from build123d import *

# Parameters (mm, degrees)
SKETCH_1_W               = 165.5
SKETCH_1_H               = 60
EXTRUDE_1_DEPTH          = 4
EXTRUDE_2_DEPTH          = 4
SKETCH_3_W               = 214.285714285
SKETCH_3_H               = 25
EXTRUDE_5_DEPTH          = 4
SKETCH_4_R               = 2.75
CUT_EXTRUDE_1_DEPTH      = 4
SKETCH_5_W               = 55
SKETCH_5_H               = 20
CUT_EXTRUDE_2_DEPTH      = 4
FILLET_1_R               = 10
SKETCH_6_W               = 186.285714285
SKETCH_6_H               = 14
CUT_EXTRUDE_3_DEPTH      = 4
SKETCH_7_R               = 1.5
CUT_EXTRUDE_4_DEPTH      = 4
FILLET_2_R               = 3
CUT_EXTRUDE_5_DEPTH      = 4
FILLET_1_OF_MIRROR_1_R   = 10
FILLET_2_OF_MIRROR_1_R   = 3
CUT_EXTRUDE_6_DEPTH      = 292.712781796
CUT_EXTRUDE_6_DEPTH_BACK = 4
SKETCH_9_W               = 205.055051827
SKETCH_9_H               = 163.821453507
CUT_EXTRUDE_7_DEPTH      = 293.240221501
SKETCH_11_W              = 207.248718004
SKETCH_11_H              = 34
EXTRUDE_6_DEPTH          = 4
SKETCH_12_W              = 22
SKETCH_12_H              = 28
EXTRUDE_7_DEPTH          = 4
SKETCH_13_R              = 2.75
CUT_EXTRUDE_8_DEPTH      = 4
EXTRUDE_8_DEPTH          = 4
FILLET_3_R               = 10
SKETCH_15_W              = 10
SKETCH_15_H              = 10
CUT_EXTRUDE_9_DEPTH      = 4
FILLET_4_R               = 2
CHAMFER_1_SIZE           = 0.5
CHAMFER_2_SIZE           = 0.5


with BuildPart() as part:
    # 草图1 → 凸台-拉伸1 (new body)
    with BuildSketch(Plane(origin=(0, 0, 0), x_dir=(0, 0, -1), z_dir=(1, 0, 0))):
        with Locations((82.75, 30)):
            Rectangle(SKETCH_1_W, SKETCH_1_H)
    extrude_1 = extrude(amount=EXTRUDE_1_DEPTH)

    # 草图2 → 凸台-拉伸2 (add)
    with BuildSketch(Plane(origin=(0, 0, -165.5), x_dir=(-1, 0, 0), z_dir=(0, 0, -1))):
        Polygon((-4, 30), (-204, 106.930925816), (-193.94769236, 133.06425915), (-4, 60), align=None)
    extrude_2 = extrude(amount=-EXTRUDE_2_DEPTH)

    # 草图3 → 凸台-拉伸5 (add)
    with BuildSketch(Plane(origin=(-9.536752084, 24.793025648, 0), x_dir=(0.9333333333333335, 0.3590109871422999, 0), z_dir=(0.3590109871422999, -0.9333333333333335, 0))):
        with Locations((121.646520091, -153)):
            Rectangle(SKETCH_3_W, SKETCH_3_H)
    extrude_5 = extrude(amount=-EXTRUDE_5_DEPTH)

    # 草图4 → 切除-拉伸1 (cut)
    with BuildSketch(Plane(origin=(4, 0, 0), x_dir=(0, 0, -1), z_dir=(1, 0, 0))):
        with Locations((50, 50)):
            Circle(SKETCH_4_R)
        with Locations((50, 20)):
            Circle(SKETCH_4_R)
    cut_extrude_1 = extrude(amount=-CUT_EXTRUDE_1_DEPTH, mode=Mode.SUBTRACT)

    # 草图5 → 切除-拉伸2 (cut)
    with BuildSketch(Plane(origin=(4, 0, 0), x_dir=(0, 0, -1), z_dir=(1, 0, 0))):
        with Locations((138, 10)):
            Rectangle(SKETCH_5_W, SKETCH_5_H)
    cut_extrude_2 = extrude(amount=-CUT_EXTRUDE_2_DEPTH, mode=Mode.SUBTRACT)

    # 圆角1
    fillet_1_edges = [part.edges().sort_by_distance(p)[0] for p in [
        (2, 20, -165.5),
        (2, 20, -110.5),
        (2, 0, -110.5),
    ]]
    fillet(fillet_1_edges, radius=FILLET_1_R - 0.0001)  # a hair under: the kernel refuses the full size

    # 草图6 → 切除-拉伸3 (cut)
    with BuildSketch(Plane(origin=(-9.536752084, 24.793025648, 0), x_dir=(0.9333333333333335, 0.35901098714229984, 0), z_dir=(0.35901098714229984, -0.9333333333333335, 0))):
        with Locations((121.646520091, -147.5)):
            Rectangle(SKETCH_6_W, SKETCH_6_H)
    cut_extrude_3 = extrude(amount=-CUT_EXTRUDE_3_DEPTH, mode=Mode.SUBTRACT)

    # 草图7 → 切除-拉伸4 (cut)
    with BuildSketch(Plane(origin=(-9.536752084, 24.793025648, 0), x_dir=(0.9333333333333335, 0.35901098714229984, 0), z_dir=(0.35901098714229984, -0.9333333333333335, 0))):
        with Locations((221.789377233, -145.5)):
            Circle(SKETCH_7_R)
        with Locations((21.789377233, -145.5)):
            Circle(SKETCH_7_R)
    cut_extrude_4 = extrude(amount=-CUT_EXTRUDE_4_DEPTH, mode=Mode.SUBTRACT)

    # 圆角2
    fillet_2_edges = [part.edges().sort_by_distance(p)[0] for p in [
        (4, 32.142857143, -140.5),
        (203.281978026, 108.797592483, -140.5),
        (16.348644692, 36.892820487, -140.5),
        (190.215311359, 103.771438663, -140.5),
    ]]
    fillet(fillet_2_edges, radius=FILLET_2_R)

    # 草图8 → 切除-拉伸5 (cut)
    with BuildSketch(Plane.XY.offset(-161.5)):
        Polygon((45.333333333, 45.899058002), (39.948168526, 59.899058002), (170.614835193, 110.160596202), (176, 96.160596202), align=None)
    cut_extrude_5 = extrude(amount=-CUT_EXTRUDE_5_DEPTH, mode=Mode.SUBTRACT)

    # 镜向1: 凸台-拉伸1, 凸台-拉伸2, 凸台-拉伸5, 切除-拉伸1, 切除-拉伸2, 切除-拉伸3, 切除-拉伸4, 切除-拉伸5 across plane
    add(extrude_1.mirror(Plane.XY))
    add(extrude_2.mirror(Plane.XY))
    add(extrude_5.mirror(Plane.XY))
    add(cut_extrude_1.mirror(Plane.XY), mode=Mode.SUBTRACT)
    add(cut_extrude_2.mirror(Plane.XY), mode=Mode.SUBTRACT)
    add(cut_extrude_3.mirror(Plane.XY), mode=Mode.SUBTRACT)
    add(cut_extrude_4.mirror(Plane.XY), mode=Mode.SUBTRACT)
    add(cut_extrude_5.mirror(Plane.XY), mode=Mode.SUBTRACT)

    # 圆角1 of 镜向1
    fillet_1_of_mirror_1_edges = [part.edges().sort_by_distance(p)[0] for p in [
        (2, 20, 165.5),
        (2, 20, 110.5),
        (2, 0, 110.5),
    ]]
    fillet(fillet_1_of_mirror_1_edges, radius=FILLET_1_OF_MIRROR_1_R - 0.0001)  # a hair under: the kernel refuses the full size

    # 圆角2 of 镜向1
    fillet_2_of_mirror_1_edges = [part.edges().sort_by_distance(p)[0] for p in [
        (4, 32.142857143, 140.5),
        (203.281978026, 108.797592483, 140.5),
        (16.348644692, 36.892820487, 140.5),
        (190.215311359, 103.771438663, 140.5),
    ]]
    fillet(fillet_2_of_mirror_1_edges, radius=FILLET_2_OF_MIRROR_1_R)

    # 草图9 → 切除-拉伸6 (cut, two sides: drawn at the far end of the back side and taken through both)
    with BuildSketch(Plane(origin=(4, 0, 0), x_dir=(0, 0, -1), z_dir=(1, 0, 0)).offset(-CUT_EXTRUDE_6_DEPTH_BACK)):
        with Locations((102.527525913, 81.910726754)):
            Rectangle(SKETCH_9_W, SKETCH_9_H)
    extrude(amount=CUT_EXTRUDE_6_DEPTH + CUT_EXTRUDE_6_DEPTH_BACK, mode=Mode.SUBTRACT)

    # 草图10 → 切除-拉伸7 (cut, through all)
    with BuildSketch(Plane.XY.offset(161.5)):
        Polygon((174.563956051, 99.893929535), (43.897289385, 49.632391335), (45.333333333, 45.899058002), (176, 96.160596202), align=None)
    extrude(amount=-CUT_EXTRUDE_7_DEPTH, mode=Mode.SUBTRACT)

    # 草图11 → 凸台-拉伸6 (add)
    with BuildSketch(Plane(origin=(-19.589059724, 50.926358981, 0), x_dir=(0.9333333333333335, 0.3590109871422999, 0), z_dir=(-0.3590109871422999, 0.9333333333333335, 0))):
        with Locations((125.165018231, -148.5)):
            Rectangle(SKETCH_11_W, SKETCH_11_H)
    extrude(amount=-EXTRUDE_6_DEPTH)

    # 草图12 → 凸台-拉伸7 (add)
    with BuildSketch(Plane(origin=(213.536752084, 82.137900168, 0), x_dir=(0, 0, -1), z_dir=(0.9333333333333338, 0.35901098714229945, 0))):
        with Locations((-154.5, 40.563956051)):
            Rectangle(SKETCH_12_W, SKETCH_12_H)
    extrude(amount=EXTRUDE_7_DEPTH)

    # 草图13 → 切除-拉伸8 (cut)
    with BuildSketch(Plane(origin=(217.270085418, 83.573944117, 0), x_dir=(0, 0, -1), z_dir=(0.9333333333333338, 0.35901098714229945, 0))):
        with Locations(Location((-155.5, 40.563956051, 0), (0, 0, 90))):
            Circle(SKETCH_13_R)
    extrude(amount=-CUT_EXTRUDE_8_DEPTH, mode=Mode.SUBTRACT)

    # 草图14 → 凸台-拉伸8 (add)
    with BuildSketch(Plane(origin=(0, 0, 131.5), x_dir=(-1, 0, 0), z_dir=(0, 0, -1))):
        Polygon((-4, 55.714285714), (-4, 60), (0, 60), (0, 133.06425915), (-193.94769236, 133.06425915), (-195.383736309, 129.330925816), align=None)
    extrude(amount=EXTRUDE_8_DEPTH)

    # 圆角3
    fillet_3_edges = [part.edges().sort_by_distance(p)[0] for p in [
        (0, 133.06425915, 129.5),
    ]]
    fillet(fillet_3_edges, radius=FILLET_3_R)

    # 草图15 → 切除-拉伸9 (cut)
    with BuildSketch(Plane.XY.offset(131.5)):
        with Locations((15, 118.06425915)):
            Rectangle(SKETCH_15_W, SKETCH_15_H)
        with Locations((27, 118.06425915)):
            Rectangle(SKETCH_15_W, SKETCH_15_H)
        with Locations((15, 106.06425915)):
            Rectangle(SKETCH_15_W, SKETCH_15_H)
        with Locations((27, 106.06425915)):
            Rectangle(SKETCH_15_W, SKETCH_15_H)
    extrude(amount=-CUT_EXTRUDE_9_DEPTH, mode=Mode.SUBTRACT)

    # 圆角4
    fillet_4_edges = [part.edges().sort_by_distance(p)[0] for p in [
        (32, 123.06425915, 129.5),
        (10, 101.06425915, 129.5),
        (32, 101.06425915, 129.5),
        (10, 123.06425915, 129.5),
    ]]
    fillet(fillet_4_edges, radius=FILLET_4_R)

    # 倒角1
    chamfer_1_edges = [part.edges().sort_by_distance(p)[0] for p in [
        (22, 118.06425915, 127.5),
        (22, 113.06425915, 129.5),
        (22, 123.06425915, 129.5),
        (32, 117.06425915, 127.5),
        (27, 113.06425915, 127.5),
        (22, 118.06425915, 131.5),
        (27, 113.06425915, 131.5),
        (32, 117.06425915, 131.5),
        (10, 107.06425915, 127.5),
        (15, 111.06425915, 127.5),
        (10, 111.06425915, 129.5),
        (10, 107.06425915, 131.5),
        (15, 111.06425915, 131.5),
        (22, 106.06425915, 127.5),
        (22, 101.06425915, 129.5),
        (27, 111.06425915, 127.5),
        (22, 111.06425915, 129.5),
        (26, 101.06425915, 127.5),
        (22, 106.06425915, 131.5),
        (26, 101.06425915, 131.5),
        (27, 111.06425915, 131.5),
        (10, 113.06425915, 129.5),
        (16, 123.06425915, 127.5),
        (15, 113.06425915, 127.5),
        (15, 113.06425915, 131.5),
        (16, 123.06425915, 131.5),
        (26, 123.06425915, 131.5),
        (26, 123.06425915, 127.5),
        (10, 117.06425915, 131.5),
        (10, 117.06425915, 127.5),
        (16, 101.06425915, 131.5),
        (16, 101.06425915, 127.5),
        (32, 107.06425915, 131.5),
        (32, 107.06425915, 127.5),
        (31.414213562, 122.478472712, 131.5),
        (31.414213562, 122.478472712, 127.5),
        (10.585786438, 122.478472712, 131.5),
        (10.585786438, 122.478472712, 127.5),
        (10.585786438, 101.650045587, 131.5),
        (10.585786438, 101.650045587, 127.5),
        (31.414213562, 101.650045587, 131.5),
        (31.414213562, 101.650045587, 127.5),
    ]]
    chamfer(chamfer_1_edges, length=CHAMFER_1_SIZE)

    # 倒角2
    chamfer_2_edges = [part.edges().sort_by_distance(p)[0] for p in [
        (203.694459728, 118.866969765, 155.5),
    ]]
    chamfer(chamfer_2_edges, length=CHAMFER_2_SIZE)


solid = part.part
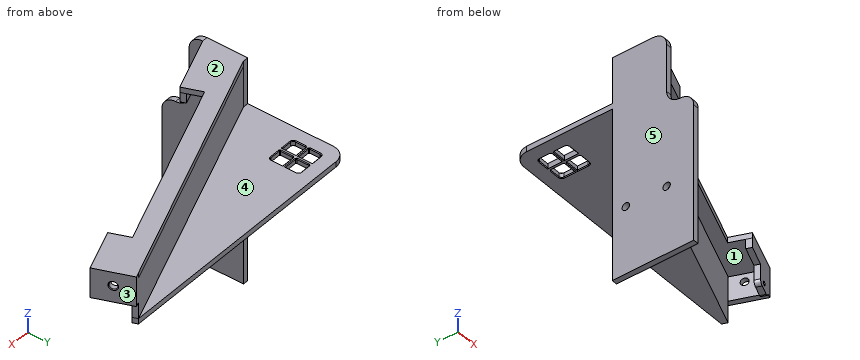
Input: part model. Units: mm. Frame: model coordinates. Face numbers are marked on the shaded views. A direction names the side the tool comes from. Round coordinates to 2 decimals unless told otherwise and drop trailing zeros. Loops run counter-clockwise (first coordinate to the right, second up) from the corner with the lowest first, then second, coordinate; pieces in that order, holes last. Notation, with made-up numbers: M -38.5,67 L -30.5,67 A22 cw -30.5,90 Z; hole C -9,-20.5 d10. An arc over 180 degrees is marked long. Answer as CSV lines item,"result". Start each with the question number.
(1) First-contact query: pin 1 (4.5 mm diameter, centred on x = 185, y = 100, fed in from -Z); pin 2 (1.5 mm diameter, centred on x = 27.5, z = 129.5, fed in from +Y); pin 3 (3.5 mm diameter, centred on x = 24.5, z = 129, fed in from -Y). Flat tips, straight axial feed; report the tip coordinate or a pass-through.
(2) Reachability of the marked faces 4 and 5 from +Z, -Z, +X, -X, +Y, -Y: full face, straight path, thin tool, end or side. Return the list, or none.
(3) Section C-C, the plane y = 63. Output: boundary loops of the cut face in (x, z).
(4) Section B-B, the plane y = 87. Output: boundary loops of the cut face in (x, z), plus the area to 3 significant figures.
(5) Section A-A, the plane z = 50. Output: boundary loops of the cut face in (x, y).
(6) Draft query along X for the marked faces 1, 2 and 3. Return one class per face: released by +X, released by -X, zero draft, split by the parting line, or undercut.
(7) Line query: line 1 (Y direction, x = 1.85, z = 50); line 2 (Z direction, x = 174, y = 101.5); line 3 (X direction, y = 41, z = 104). Output: solid intervals per line, ascending. Write a range as [from, to].
Values found:
1,pin 1,"stops at z = 154.5"
1,pin 2,"stops at y = 133.06"
1,pin 3,"stops at y = 62.93"
2,face 4,"+Z, -X, +Y"
2,face 5,"+Z, -Z, -X, +Y, -Y"
3,outline,"M 0,127.5 L 22.94,127.5 L 22.94,161.5 L 48.01,161.5 L 48.01,165.5 L 11.8,165.5 L 11.8,131.5 L 0,131.5 Z"
4,outline,"M 0,127.5 L 85.33,127.5 L 85.33,161.5 L 110.4,161.5 L 110.4,165.5 L 74.19,165.5 L 74.19,131.5 L 0,131.5 Z"
4,area,"820 mm²"
5,outline,"M 0,0 L 4,0 L 4,17.25 L 0,17.25 Z; M 0,22.75 L 4,22.75 L 4,47.25 L 0,47.25 Z; M 0,52.75 L 4,52.75 L 4,60 L 0,60 Z"
6,face 1,"undercut"
6,face 2,"zero draft"
6,face 3,"released by +X"
7,line 1,"y = [0, 17.25], [22.75, 47.25], [52.75, 60]"
7,line 2,"z = [161.5, 165.5]"
7,line 3,"x = [0, 4]"
